Check sheet for the modelled part. Datum: model origin and axes. Units: mm. A direction names the side the tool comes from. Give positions to 0.01 mm unless a question says otherwise; leave off trailing zeros. Order: outer loops, then holes, each group sorted by start corner. A loop starts at its lowest first (then second) coordinate and runs counter-clockwise, first axis right, second up.
```python
from build123d import *

# Parameters (mm, degrees)
SKETCH1_W          = 20
SKETCH1_H          = 20
EXTRUDE1_DEPTH     = 3.5
SKETCH2_W          = 20
SKETCH2_H          = 3.5
EXTRUDE2_DEPTH     = 16.5
EXTRUDE3_DEPTH     = 2.9
EXTRUDE4_DEPTH     = 2.9
CUT_EXTRUDE1_REACH = 5.5
CUT_EXTRUDE2_REACH = 5.5


with BuildPart() as part:
    # Sketch1 → Extrude1 (new body)
    with BuildSketch(Plane.XY):
        with Locations((10, 10)):
            Rectangle(SKETCH1_W, SKETCH1_H)
    extrude(amount=EXTRUDE1_DEPTH)

    # Sketch2 → Extrude2 (add)
    with BuildSketch(Plane.XY.offset(3.5)):
        with Locations((10, 1.75)):
            Rectangle(SKETCH2_W, SKETCH2_H)
    extrude(amount=EXTRUDE2_DEPTH)

    # Sketch5 → Extrude3 (add)
    with BuildSketch(Plane(origin=(20, 0, 0), x_dir=(0, 0, -1), z_dir=(1, 0, 0))):
        Polygon((-3.5, 20), (-20, 3.5), (-3.5, 3.5), align=None)
    extrude(amount=-EXTRUDE3_DEPTH)

    # Sketch6 → Extrude4 (add)
    with BuildSketch(Plane.ZY):
        Polygon((3.5, 20), (20, 3.5), (3.5, 3.5), align=None)
    extrude(amount=-EXTRUDE4_DEPTH)

    # Sketch7 → Cut-Extrude1 (cut, up to next)
    with BuildSketch(Plane(origin=(0, 3.5, 0), x_dir=(1, 0, 0), z_dir=(0, 1, 0)), mode=Mode.PRIVATE) as cut_extrude1_sk1:
        with BuildLine():
            Line((7.45, -14), (7.45, -9.5))
            ThreePointArc((7.45, -9.5), (10, -6.95), (12.55, -9.5))
            Line((12.55, -9.5), (12.55, -14))
            ThreePointArc((12.55, -14), (10, -16.55), (7.45, -14))
        make_face()
    cut_extrude1_tool1 = extrude(cut_extrude1_sk1.sketch, amount=-CUT_EXTRUDE1_REACH, mode=Mode.PRIVATE) & part.part
    add(cut_extrude1_tool1.solids().sort_by_distance((10, 3.5, 11.75))[0], mode=Mode.SUBTRACT)

    # Sketch8 → Cut-Extrude2 (cut, up to next)
    with BuildSketch(Plane(origin=(0, 0, 3.5), x_dir=(-1, 0, 0), z_dir=(0, 0, 1)), mode=Mode.PRIVATE) as cut_extrude2_sk1:
        with BuildLine():
            Line((-12.55, -14), (-12.55, -9.5))
            ThreePointArc((-12.55, -9.5), (-10, -6.95), (-7.45, -9.5))
            Line((-7.45, -9.5), (-7.45, -14))
            ThreePointArc((-7.45, -14), (-10, -16.55), (-12.55, -14))
        make_face()
    cut_extrude2_tool1 = extrude(cut_extrude2_sk1.sketch, amount=-CUT_EXTRUDE2_REACH, mode=Mode.PRIVATE) & part.part
    add(cut_extrude2_tool1.solids().sort_by_distance((10, 11.75, 3.5))[0], mode=Mode.SUBTRACT)


solid = part.part
```
(1) Sectioned sample at C-C (x = 10). Enter the section's corners in (y, z), plus the area to 4 significant figures.
(2) Tool access check on faces 4 (the face through (7.45, 2, 12)), 5 (the face through (2.9, 8, 8)), 6 (the face through (9.94, 16.55, 1.77)). Record the directions out of +Z, -Z, +X, -X, +Y, -Y that give a thin tool (end or side, any length) a straight path to the whole face; none if there is none.
(3) Sectioned sample at B-B (y = 7.25). Enter the section's corners in (x, z).
(4) Sectioned sample at A-A (z = 10). Enter the section's corners in (x, y), plus the area to 3 significant figures.
(5) Sectioned sample at D-D (z = 18.5). Enter the section's corners in (x, y), plus the area to 3 significant figures.
(6) Release check for a two-part mould opening along Z. For faces 1 (the face through (10.06, 1.77, 16.55)), 2 (the face through (17.1, 8, 8)), 3 (the face through (10, 2, 20)) record: released by +Z, released by -Z, zero draft, split by the parting line, or undercut.
(7) Thickness scan on L1, parallel to X at y = 13.25, z = 5; L2, parallel to Z at x = 3.25, y = 6. Record the ranges inside material, lowest first.
(8) Go/stop test with flat-tipped pins: P1, Ø2, axis at x = 16.5, z = 10.5, coming from the +Y side; P2, Ø3, axis at x = 15, z = 11, coming from the +Y side; P3, Ø1, axis at x = 2.5, z = 9, coming from the +Y side. Record where each tip stops, or that it passes through.
Values follow:
1. outline: (0, 0) - (6.95, 0) - (6.95, 3.5) - (3.5, 3.5) - (3.5, 6.95) - (0, 6.95) - close; (0, 16.55) - (3.5, 16.55) - (3.5, 20) - (0, 20) - close; (16.55, 0) - (20, 0) - (20, 3.5) - (16.55, 3.5) - close
1. area: 60.55 mm2
2. face 4: +Y, -Y
2. face 5: +Z, +Y
2. face 6: +Z, -Z
3. outline: (0, 0) - (8.8, 0) - (8.8, 3.5) - (2.9, 3.5) - (2.9, 16.25) - (0, 16.25) - close; (11.2, 0) - (20, 0) - (20, 16.25) - (17.1, 16.25) - (17.1, 3.5) - (11.2, 3.5) - close
4. outline: (0, 0) - (7.45, 0) - (7.45, 3.5) - (2.9, 3.5) - (2.9, 13.5) - (0, 13.5) - close; (12.55, 0) - (20, 0) - (20, 13.5) - (17.1, 13.5) - (17.1, 3.5) - (12.55, 3.5) - close
4. area: 110 mm2
5. outline: (0, 0) - (20, 0) - (20, 5) - (17.1, 5) - (17.1, 3.5) - (2.9, 3.5) - (2.9, 5) - (0, 5) - close
5. area: 78.7 mm2
6. face 1: undercut
6. face 2: zero draft
6. face 3: released by +Z
7. L1: x = 0 to 2.9, 17.1 to 20
7. L2: z = 0 to 3.5
8. P1: stops at y = 13.8
8. P2: stops at y = 3.5
8. P3: stops at y = 15
